Here's how the part is built. I have some questions about the finished solid (model axes, mm). Face numbers are marked on the shaded views. A direction names the side the tool comes from. Coordinates: 2 decimals unless noted, no trailing zeros. Loops run counter-clockwise (first coordinate to the right, second up) from the corner with the lowest first, then second, coordinate; pieces in that order, holes last. Notation, with made-up numbers: (-22, -38) - (18, -38) arc R22 ccw to (18, -7) - close; hole circle Ø1 at (-15, 47). An arc over 180 degrees is marked (long way). Use a Markdown table: item, result.
```python
from build123d import *

# Parameters (mm, degrees)
SKETCH1_R           = 17.5
BOSS_EXTRUDE1_DEPTH = 12
SKETCH2_R           = 10
BOSS_EXTRUDE2_DEPTH = 20
FILLET1_R           = 1


with BuildPart() as part:
    # Sketch1 → Boss-Extrude1 (new body)
    with BuildSketch(Plane(origin=(0, 0, 0), x_dir=(1, 0, 0), z_dir=(0, 1, 0))):
        Circle(SKETCH1_R)
    extrude(amount=BOSS_EXTRUDE1_DEPTH)

    # Sketch2 → Boss-Extrude2 (add)
    with BuildSketch(Plane.XZ):
        Circle(SKETCH2_R)
    extrude(amount=BOSS_EXTRUDE2_DEPTH)

    # Fillet1
    fillet1_edges = [part.edges().sort_by_distance(p)[0] for p in [
        (-17.5, 0, 0),
        (-17.5, 12, 0),
        (-10, 0, 0),
        (-10, -20, 0),
    ]]
    fillet(fillet1_edges, radius=FILLET1_R)


solid = part.part
```
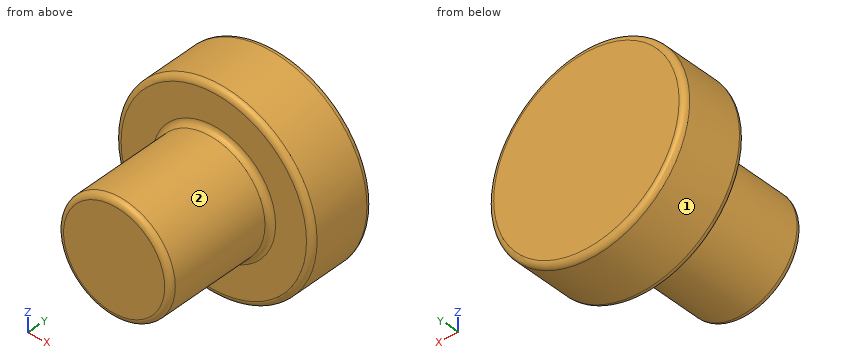
Q1. I want a section at A-A, the plane x = 0. Write out the boundary of the cut face in (y, z).
Check values:
| item | result |
|---|---|
| outline | (-20, -9) arc R1 ccw to (-19, -10) - (-1, -10) arc R1 cw to (0, -11) - (0, -16.5) arc R1 ccw to (1, -17.5) - (11, -17.5) arc R1 ccw to (12, -16.5) - (12, 16.5) arc R1 ccw to (11, 17.5) - (1, 17.5) arc R1 ccw to (0, 16.5) - (0, 11) arc R1 cw to (-1, 10) - (-19, 10) arc R1 ccw to (-20, 9) - close |
Q2. Please list where these lines run through material, in increasing order: L1, parallel to Y at x = -2.5, z = -12; L2, parallel to Z at x = -5.5, y = -16; L3, parallel to X at y = -4, z = -4.5. Write a range as from..to.
Check values:
| item | result |
|---|---|
| L1 | 0..12 |
| L2 | -8.35..8.35 |
| L3 | -8.93..8.93 |
Q3. Will these pins go through, and if not, where does the flat tip stop? P1, Ø12, axis at x = 5.5, y = -8, coming from the +Z side; P2, Ø1, axis at x = 2, y = -9, coming from the -Z side; P3, Ø3, axis at y = 5.5, z = -11, coming from the +X side.
Check values:
| item | result |
|---|---|
| P1 | z = 10 |
| P2 | z = -9.89 |
| P3 | x = 14.7 |
Q4. Which directions (+Z, -Z, +X, -X, +Y, -Y) give clear straight access to the entire face, cutting with the end or side of a thin tool? Please do the marked faces 1 and 2.
Check values:
| item | result |
|---|---|
| face 1 | +Y, -Y |
| face 2 | -Y |
Q5. I want a section at C-C, the plane y = -14.5. Write out the boundary of the cut face in (x, z).
Check values:
| item | result |
|---|---|
| outline | circle Ø20 at (0, 0) |
Q6. I want a section at B-B, the plane z = 0. Write out the boundary of the cut face in (x, y).
Check values:
| item | result |
|---|---|
| outline | (-17.5, 1) arc R1 ccw to (-16.5, 0) - (-11, 0) arc R1 cw to (-10, -1) - (-10, -19) arc R1 ccw to (-9, -20) - (9, -20) arc R1 ccw to (10, -19) - (10, -1) arc R1 cw to (11, 0) - (16.5, 0) arc R1 ccw to (17.5, 1) - (17.5, 11) arc R1 ccw to (16.5, 12) - (-16.5, 12) arc R1 ccw to (-17.5, 11) - close |
